from build123d import *

# Parameters (mm, degrees)
F0_W     = 5.387183
F0_H     = 0.69484
F1_DEPTH = 9
F2_R     = 3


with BuildPart() as f1:
    # F0 (on Top) → F1 (new body)
    with BuildSketch(Plane.XY):
        with BuildLine():
            ThreePointArc((-1.662956, 5.542424), (1.030635, 4.737264), (3.724227, 5.542424))
            Line((3.724227, 5.542424), (-1.662956, 5.542424))
        make_face()
        with Locations((1.030636, 5.889844)):
            Rectangle(F0_W, F0_H)
        with BuildLine():
            Line((3.724227, 6.237264), (3.724227, 11.237264))
            Line((3.724227, 11.237264), (-21.275773, 11.237264))
            Line((-21.275773, 11.237264), (-21.275773, -12.762736))
            Line((-21.275773, -12.762736), (3.724227, -12.762736))
            Line((3.724227, -12.762736), (3.724227, -7.762736))
            Line((3.724227, -7.762736), (-16.275773, -7.762736))
            Line((-16.275773, -7.762736), (-16.275773, 5.487264))
            ThreePointArc((-16.275773, 5.487264), (-16.806103, 6.767594), (-15.525773, 6.237264))
            Line((-15.525773, 6.237264), (-1.662956, 6.237264))
            Line((-1.662956, 6.237264), (3.724227, 6.237264))
        make_face()
    extrude(amount=F1_DEPTH)

    # F2
    f2_edges = [f1.edges().sort_by_distance(p)[0] for p in [
        (-21.275773, 11.237264, 4.5),
        (-21.275773, -12.762736, 4.5),
        (3.724227, 11.237264, 4.5),
        (3.724227, -12.762736, 4.5),
    ]]
    fillet(f2_edges, radius=F2_R)


solid = f1.part
Geometry: final body of the model. Coordinates: model frame, mm. A direction names the side the tool comes from. Round coordinates to 2 decimals unless told otherwise and drop trailing zeros. Order: outer loops, then holes, each group sorted by start corner. A loop starts at its lowest first (then second) coordinate and runs counter-clockwise, first axis right, second up.
Q1. Access query for faces 5 (the face through (3.724, -9, 4)), 6 (the face through (-9, 6.237, 4)). Directions: +Z, -Z, +X, -X, +Y, -Y. A direction counts if a zero-diameter tool reaches every point of the face in a straight line with its end or side. Return the directions, or none.
Result sheet:
face 5: +Z, -Z, +X, +Y, -Y
face 6: +Z, -Z
Q2. Material intervals for probe 1 along Y at (x, z) = (-2.5, 8); probe 2 along X at (y, z) = (4.25, 5.25); probe 3 along Y at (x, z) = (-16.5, 3.75), sorted ascending.
Result sheet:
probe 1: y = -12.76 to -7.76, 6.24 to 11.24
probe 2: x = -21.28 to -16.28
probe 3: y = -12.76 to 5.52, 6.95 to 11.24
Q3. Section C-C, the plane x = -0.5. Output: boundary loops of the cut face in (y, z), and give its area (3 significant figures).
Result sheet:
outline: (-12.76, 0) - (-7.76, 0) - (-7.76, 9) - (-12.76, 9) - close; (4.98, 0) - (11.24, 0) - (11.24, 9) - (4.98, 9) - close
area: 101 mm2
Q4. Section B-B, the plane z = 4. Output: boundary loops of the cut face in (x, y), and give its area (3 significant figures).
Result sheet:
outline: (-21.28, -9.76) arc R3 ccw to (-18.28, -12.76) - (0.72, -12.76) arc R3 ccw to (3.72, -9.76) - (3.72, -7.76) - (-16.28, -7.76) - (-16.28, 5.49) arc R0.75 cw (long way) to (-15.53, 6.24) - (-1.66, 6.24) - (-1.66, 5.54) arc R4.91 ccw to (3.72, 5.54) - (3.72, 8.24) arc R3 ccw to (0.72, 11.24) - (-18.28, 11.24) arc R3 ccw to (-21.28, 8.24) - close
area: 318 mm2
Q5. Section A-A, the plane x = -4.25. Output: boundary loops of the cut face in (y, z).
Result sheet:
outline: (-12.76, 0) - (-7.76, 0) - (-7.76, 9) - (-12.76, 9) - close; (6.24, 0) - (11.24, 0) - (11.24, 9) - (6.24, 9) - close
Q6. Mould query, pull axis Y, two halves, no side actions, for faces 1 (the face through (2.9, 10.3, 4.6)), 2 (the face through (3.724, 7, 4)), 3 (the face through (-16.823, 6.75, 4.437)), 4 (the face through (-6, -7.763, 4)). Classes: released by +Y, released by -Y, zero draft, split by the parting line, or undercut.
Result sheet:
face 1: released by +Y
face 2: zero draft
face 3: undercut
face 4: undercut
Q7. Pin query (flat end, axial travel): pin 1 (2.5 mm diameter, centred on x = -16.28, y = 6.24, fed in from +Z); pin 2 (4 mm diameter, centred on y = 3.5, z = 5.5, fed in from +X); pin 3 (1 mm diameter, centred on x = -3.5, y = 4, fed in from +Z). Return the tip coordinate at first contact, or that it passes through.
Result sheet:
pin 1: stops at z = 9
pin 2: stops at x = 3.66
pin 3: passes through
Q8. Section D-D, the plane y = -1.5. Output: boundary loops of the cut face in (x, z), and give its area (3 significant figures).
Result sheet:
outline: (-21.28, 0) - (-16.28, 0) - (-16.28, 9) - (-21.28, 9) - close
area: 45.0 mm2
